Check sheet for the modelled part. Datum: model origin and axes. Units: mm. A direction names the side the tool comes from. Give positions to 0.01 mm unless a question says otherwise; leave off trailing zeros. Write each loop counter-clockwise with the first axis right and the second up, starting at its lowest first coordinate (ties: lowest second). Pieces come first, ordered by that corner, then holes. Notation, with made-up numbers: M 45.5,59.5 L 81.5,59.5 A10 cw 81.5,66.5 Z; hole C -28.75,69 d9. An arc over 180 degrees is marked long. Write item = value, one per line. Start each with the question number.
1) Scan lines: line 1 along X through (y, z) = (-13.5, 44); line 2 along X through (y, z) = (-11, 28.5); line 3 along Y through (x, z) = (6.25, 44). Record each from-to range of solid material in increasing order. Write a range as [from, to].
2) Mould release check, pull along Y, two halves, no side actions. Record for faces 1 (the flat face through (-12.019, -11, 35)), 2 (the flat face through (12, -14.258, 35)), 3 (the cylindrical face through (0, -20, 35)): released by +Y, released by -Y, zero draft, split by the parting line, or undercut.
3) Cross-section at A-A, the plane z = 5.5. Record the cut outline in (x, y), plus the area to 3 significant figures.
4) Access from +Z, -Z, +X, -X, +Y, -Y to the whole of each face (thin tool, end or side, straight path). Record for faces 4 (the flat face through (12.019, -11, 35)), 5 (the flat face through (-10.519, -13, 35)), 6 (the flat face through (10.519, -13, 35)).
5) Go/stop test with flat-tipped pins: pin 1 (10 mm diameter, centred on x = 5, z = 29, fed in from -Y); pin 2 (1.2 mm diameter, centred on y = -13, z = 21.5, fed in from +X); pin 3 (0.8 mm diameter, centred on x = 11.5, z = 49, fed in from -Y); pin 4 (0.8 mm diameter, centred on y = -12.5, z = 47.5, fed in from -X). Record where each tip stops, or that it passes through.
6) Cross-section at C-C, the plane x = -5.5. Record the cut outline in (y, z), plus the area to 3 significant figures.
7) Cross-section at B-B, the plane y = -12.5. Record the cut outline in (x, z), plus the area to 3 significant figures.
Autodesk Inventor part; units mm, degrees
ref_plane "YZ Plane" through (0, 0, 0) normal (1, 0, 0) x (0, 1, 0)
ref_plane "XZ Plane" through (0, 0, 0) normal (0, 1, 0) x (-1, 0, 0)
ref_plane "XY Plane" through (0, 0, 0) normal (0, 0, 1) x (1, 0, 0)
sketch "Эскиз1" plane through (0, 0, 0) normal (0, 0, 1) x (1, 0, 0)
  arc A0 (-14.0253, -14.258) -> (14.0253, -14.258) centre (0, 0) ccw
  line L0 (0, 0) -> (0, -20) construction
  line L1 (-10.5193, -14.258) -> (-10.5193, -11.758)
  line L2 (-10.5193, -11.758) -> (-12.0193, -11.758)
  line L3 (-12.0193, -11.758) -> (-12.0193, -10.258)
  line L4 (-12.0193, -10.258) -> (0, -10.258)
  line L5 (10.5193, -14.258) -> (10.5193, -11.758)
  line L6 (10.5193, -11.758) -> (12.0193, -11.758)
  line L7 (12.0193, -11.758) -> (12.0193, -10.258)
  line L8 (12.0193, -10.258) -> (0, -10.258)
  line L9 (-14.0253, -14.258) -> (-10.5193, -14.258)
  line L10 (10.5193, -14.258) -> (14.0253, -14.258)
  dimension "d0" = 40
  dimension "d2" = 2.5
  dimension "d3" = 1.5
  dimension "d4" = 1.5
  dimension "d5" = 3.506
extrude "Выдавливание1" add sketch "Эскиз1" along normal blind 70
properties part number "cap"
Reply:
q1.line_1 = [-10.52, 10.52]
q1.line_2 = [-12.02, 12.02]
q1.line_3 = [-19, -10.26]
q2.face_1 = zero draft
q2.face_2 = undercut
q2.face_3 = released by -Y
q3.outline = M -14.03,-14.26 A20 ccw 14.03,-14.26 L 10.52,-14.26 L 10.52,-11.76 L 12.02,-11.76 L 12.02,-10.26 L -12.02,-10.26 L -12.02,-11.76 L -10.52,-11.76 L -10.52,-14.26 Z
q3.area = 200 mm2
q4.face_4 = +Z, -Z, +X, +Y
q4.face_5 = +Z, -Z, -X
q4.face_6 = +Z, -Z, +X
q5.pin_1 = -20
q5.pin_2 = 10.52
q5.pin_3 = -16.64
q5.pin_4 = -10.52
q6.outline = M -19.23,0 L -10.26,0 L -10.26,70 L -19.23,70 Z
q6.area = 628 mm2
q7.outline = M -10.52,0 L 10.52,0 L 10.52,70 L -10.52,70 Z
q7.area = 1,470 mm2
